Model file for the job. Use its own axes, mm. A direction names the side the tool comes from. Coordinates: 2 decimals unless noted, no trailing zeros. Order: outer loops, then holes, each group sorted by start corner. A loop starts at its lowest first (then second) coordinate and runs counter-clockwise, first axis right, second up.
from build123d import *

# Parameters (mm, degrees)
F0_W     = 150
F0_H     = 150
F1_DEPTH = 10
F2_R     = 15.875
F2_R_2   = 13.375
F3_DEPTH = 250
F4_R     = 7.5
F5_DEPTH = 50
F6_R     = 7.5
F7_DEPTH = 50
F9_DEPTH = 30


# Not quite as in the source:
# - a feature names something its author has since deleted; it is built from what else it names


with BuildPart() as f1:
    # F0 (on Top) → F1 (new body)
    with BuildSketch(Plane.XY):
        Rectangle(F0_W, F0_H)
    extrude(amount=-F1_DEPTH)

    # F2 (on face) → F3 (join)
    with BuildSketch(Plane(origin=(0, 0, -10), x_dir=(1, 0, 0), z_dir=(0, 0, -1))):
        Circle(F2_R)
        Circle(F2_R_2, mode=Mode.SUBTRACT)
    extrude(amount=F3_DEPTH)

    # F4 (on Front) → F5 (join, symmetric)
    with BuildSketch(Plane.XZ):
        with Locations((0, -210)):
            Circle(F4_R)
    extrude(amount=F5_DEPTH, both=True)

    # F6 (on Right) → F7 (join, symmetric)
    with BuildSketch(Plane.YZ):
        with Locations((0, -190)):
            Circle(F6_R)
    extrude(amount=F7_DEPTH, both=True)

    # F8 (on Front) → F9 (join, symmetric)
    with BuildSketch(Plane.XZ):
        with BuildLine():
            Line((-10.5, 8), (-10.5, 0))
            Line((-10.5, 0), (-8, 0))
            Line((-8, 0), (-8, 8))
            ThreePointArc((-8, 8), (-5.6568542495, 13.6568542495), (0, 16))
            ThreePointArc((0, 16), (5.6568542495, 13.6568542495), (8, 8))
            Line((8, 8), (8, 0))
            Line((8, 0), (10.5, 0))
            Line((10.5, 0), (10.5, 8))
            ThreePointArc((10.5, 8), (7.4246212025, 15.4246212025), (0, 18.5))
            ThreePointArc((0, 18.5), (-7.4246212025, 15.4246212025), (-10.5, 8))
        make_face()
    extrude(amount=F9_DEPTH, both=True)


solid = f1.part
Q1. Probe line 1 (Y direction, x = 0, z = -62.5) (3 decimals); line 2 (Z direction, x = 27, y = -1). List the from-to ranges inside material, lowest first.
Established:
line 1: y = -15.875 to -13.375, 13.375 to 15.875
line 2: z = -197.43 to -182.57, -10 to 0
Q2. Which spindle directions (+Z, -Z, +X, -X, +Y, -Y) get a long thin tool onto all of the face, cutting with end or side? Do faces 1 (the face through (7.154, 31.743, -207.747)), 2 (the face through (10.5, 0, 4)), 3 (the face through (0, 50, -210)), 4 (the face through (-0.976, -32.248, -202.564)). Say none if no direction does.
Established:
face 1: +Y
face 2: +Z, +X, +Y, -Y
face 3: -Z, +X, -X, +Y
face 4: -Y
Q3. Cut at C-C, the plane y = -43. List the corners of the cut face in (x, z), plus the area to 3 significant figures.
Established:
outline: (-75, -10) - (75, -10) - (75, 0) - (-75, 0) - close; circle Ø15 at (0, -210)
area: 1,680 mm2
Q4. Drop flat-ended pins along their axis: P1, Ø15, axis at x = -5, z = 11, coming from the -Y side; P2, Ø2.5, axis at y = 4, z = 4.5, coming from the +X side; P3, Ø4, axis at x = 50.5, y = -40.5, coming from the +Z side; P4, Ø8, axis at x = -21.5, z = -155.5, coming from the -Y side. Give the stop position or say it passes through.
Established:
P1: stops at y = -30
P2: stops at x = 10.5
P3: stops at z = 0
P4: passes through
Q5. Cut at D-D, the plane z = -18. List the corners of the cut face in (x, y) (3 decimals).
Established:
outline: circle Ø31.75 at (0, 0); hole circle Ø26.75 at (0, 0)
Q6. Mould opens along X. For faces 5 (the face through (0.2, -5.5, -184.9)), 6 (the face through (-50, 0, -190)), 7 (the face through (-1, -75, -5)) say: pulls with the +X half, pulls with the -X half, needs draft (parallel to the pull), parting line crosses it, or undercut.
Established:
face 5: undercut
face 6: pulls with the -X half
face 7: needs draft
Q7. Cut at B-B, the plane x = -36. List the corners of the cut face in (y, z).
Established:
outline: (-75, -10) - (75, -10) - (75, 0) - (-75, 0) - close; circle Ø15 at (0, -190)
Q8. Cut at A-A, the plane y = -22. List the corners of the cut face in (x, z).
Established:
outline: (-75, -10) - (75, -10) - (75, 0) - (10.5, 0) - (10.5, 8) arc R10.5 ccw to (-10.5, 8) - (-10.5, 0) - (-75, 0) - close; circle Ø15 at (0, -210); hole (-8, 0) - (8, 0) - (8, 8) arc R8 ccw to (-8, 8) - close
